Job drawing, mm, ordinate dimensions from the low corner. One solid piece. Round coordinates to 2 decimals unless told otherwise and drop trailing zeros. Loops run counter-clockwise (first coordinate to the right, second up) from the corner with the lowest first, then second, coordinate; pieces in that order, holes last. Notation, with made-up numbers: M 71,87 L 104,87 A33 ccw 104,124 Z; hole C -37,32.5 d1. An arc over 180 degrees is marked long. Put each result on its own line as item: value. Start each with the question number.
1) Slice it at A-A on z = 5.75. Give the cut face in (x, y).
2) Slice it at B-B on y = 8.5. Give the cut face in (x, z).
3) Probe line 1 along Y through (x, z) = (8, 14.5); line 2 along Y through (x, z) = (36.5, 3.5); line 3 along X through (y, z) = (12, 7.5). List the from-to ranges inside material, lowest first.
4) Drop flat-ended pins along their axis: pin 1 Ø6 at (y, z) = (9, 3.5) entering from -X; pin 2 Ø5 at (y, z) = (30.5, 6) entering from +X; pin 3 Ø4 at (y, z) = (8, 14.5) entering from +X. Give the stop position or say it passes through.
5) Slice it at C-C on x = 21. Give the cut face in (y, z).
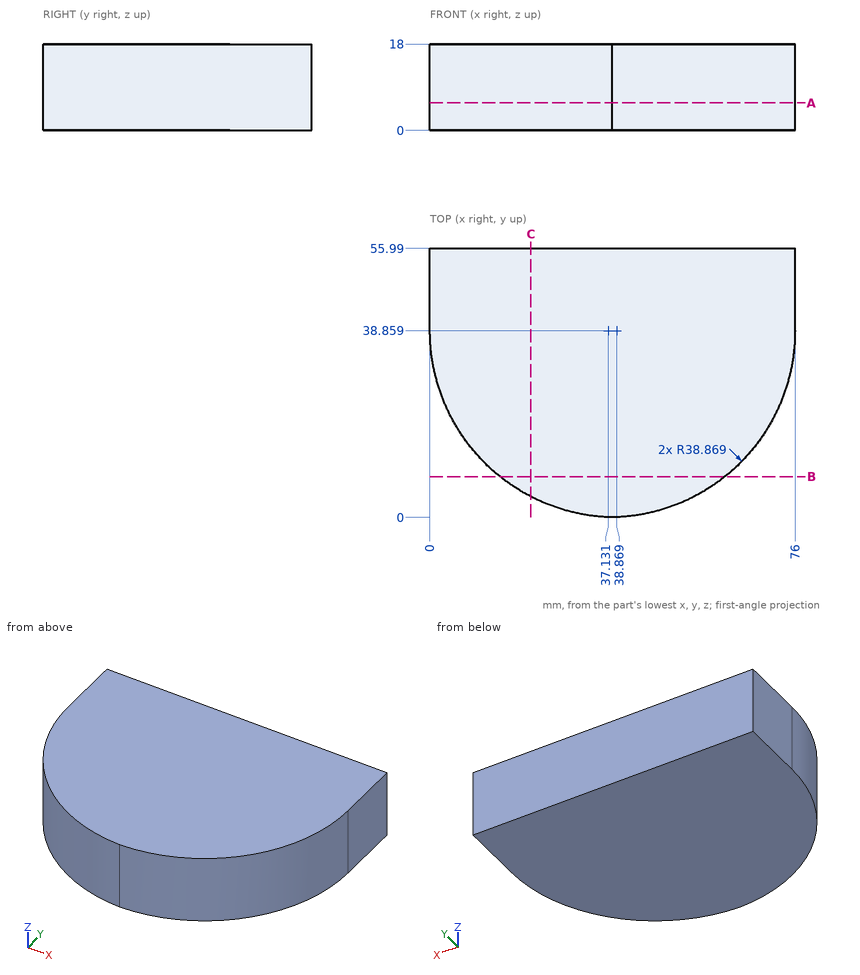
Recorded:
1. outline: M 0,38.86 A38.87 ccw 38,0 A38.87 ccw 76,38.86 L 76,55.99 L 0,55.99 Z
2. outline: M 14.6,0 L 61.4,0 L 61.4,18 L 14.6,18 Z
3. line 1: y = 15.24 to 55.99
3. line 2: y = 0.06 to 55.99
3. line 3: x = 10.77 to 65.23
4. pin 1: stops at x = 10.77
4. pin 2: stops at x = 75.56
4. pin 3: stops at x = 63.17
5. outline: M 4.34,0 L 55.99,0 L 55.99,18 L 4.34,18 Z
